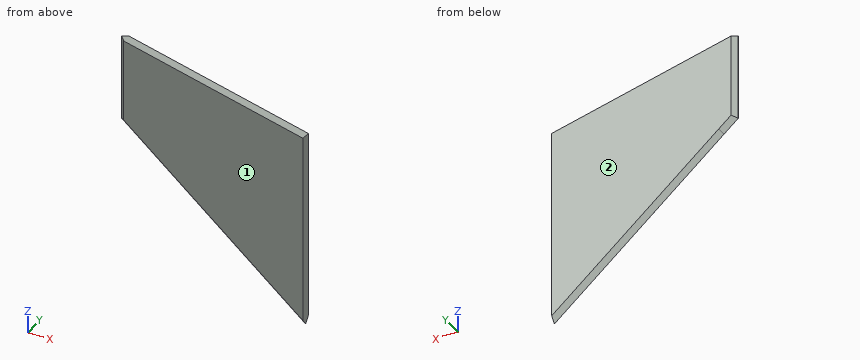
Autodesk Inventor part; units mm, degrees
ref_plane "YZ Plane" through (0, 0, 0) normal (1, 0, 0) x (0, 1, 0)
ref_plane "XZ Plane" through (0, 0, 0) normal (0, 1, 0) x (-1, 0, 0)
ref_plane "XY Plane" through (0, 0, 0) normal (0, 0, 1) x (1, 0, 0)
sketch "스케치1" plane through (0, 0, 0) normal (0, 1, 0) x (-1, 0, 0)
  line L0 (0, 0) -> (100, 0)
  line L1 (100, 0) -> (100, -130)
  line L2 (100, -130) -> (0, -130)
  line L3 (0, -130) -> (0, 0)
  line L4 (0, -130) -> (92.3211, -52.5334)
  line L5 (0, -130) -> (120.5166, -130) construction
  line L6 (92.3211, -52.5334) -> (100, -46.09)
  line L7 (100, 0) -> (0, -24.6121)
  dimension "d0" = 100
  dimension "d1" = 130
  dimension "d2" = 40
extrude "돌출1" add sketch "스케치1" along normal blind 5 contours L1 L6 L4 L3 L7
chamfer "모따기1" distance 2.5 angle 45 4 edges at (-46.1605, 5, -91.2667) (-46.1605, 0, -91.2667) (-100, 5, -23.045) (-100, 0, -23.045)
properties part number "날개1"
Work out the finished part from the listing and answer in its coordinate system (mm). Face numbers are marked on the shaded views. Coordinates: 2 decimals unless noted, no trailing zeros. Write each loop counter-clockwise with the first axis right and the second up, starting at its lowest first coordinate (ties: lowest second). Pieces come first, ordered by that corner, then holes.
Q1. Determine the mould class of the marked faces 1 and 2 for opening direction Y: released by +Y, released by -Y, zero draft, split by the parting line, or undercut.
Q2. Find the intervals of material crossed by line 1 (X direction, y = 4.7, z = -117); line 2 (Z direction, x = -84.5, y = 3.05); line 3 (Z direction, x = -48, y = 4.3), in increasing order.
Q3. A cutting plane is placed at C-C, the plane y = 3.3. Give the vertices of the cut face in (x, z), then the cut area to 3 significant figures.
Findings below:
1. face 1: released by -Y
1. face 2: released by +Y
2. line 1: x = -12.07 to 0
2. line 2: z = -58.38 to -3.81
2. line 3: z = -87.37 to -12.8
3. outline: (-99.2, -45.72) - (-91.81, -51.92) - (0, -128.96) - (0, -24.61) - (-99.2, -0.2) - close
3. area: 7,430 mm2
